Verification items for this drawing (mm, ordinates from the low corner). A direction names the side the tool comes from. Coordinates: 2 decimals unless noted, no trailing zeros. Order: outer loops, then holes, each group sorted by start corner. A loop starts at its lowest first (then second) coordinate and runs counter-clockwise, first axis right, second up. Notation, with made-up numbers: (-29, -5.75) - (-8, -5.75) arc R30 cw to (-8, 32.25) - close; hole circle Ø4 at (-24.5, 65). An arc over 180 degrees is marked (long way). Use CSV: the item, a comma, the result in double quotes. Start each with the question number.
1) Draft check along X on the marked faces 3, 4 and 5. Enter one of: released by +X, released by -X, zero draft, split by the parting line, or undercut.
2) Depth check by flat-ended pin: P1, Ø2.5, axis at y = 13.5, z = 11, coming from the -X side; P2, Ø5, axis at x = 10.5, y = 13, coming from the +Z side; P3, Ø1, axis at x = 16, y = 9, coming from the +Z side; P4, Ø2, axis at x = 18, z = 9, coming from the -Y side. Enter the tip coordinate at first touch or a pass-through.
3) Thickness scan on probe 1 along Y at (x, z) = (23.75, 7.5); probe 2 along Z at (x, y) = (23.75, 7.4); probe 3 along Y at (x, z) = (25, 7.75) (1 decimal). Record the ranges inside material, lowest first. Write a range as [from, to].
4) Sectioned sample at B-B, the plane z = 7.75. Record the cut outline in (x, y), and give its area (3 significant figures).
5) Tool access check on the marked faces 1 and 2. Record the directions out of +Z, -Z, +X, -X, +Y, -Y that give a thin tool (end or side, any length) a straight path to the whole face; none if there is none.
6) Sectioned sample at D-D, the plane z = 11.75. Record the cut outline in (x, y).
7) Sectioned sample at A-A, the plane x = 23.75. Record the cut outline in (y, z), and give its area (3 significant figures).
8) Sectioned sample at C-C, the plane y = 18.5. Record the cut outline in (x, z).
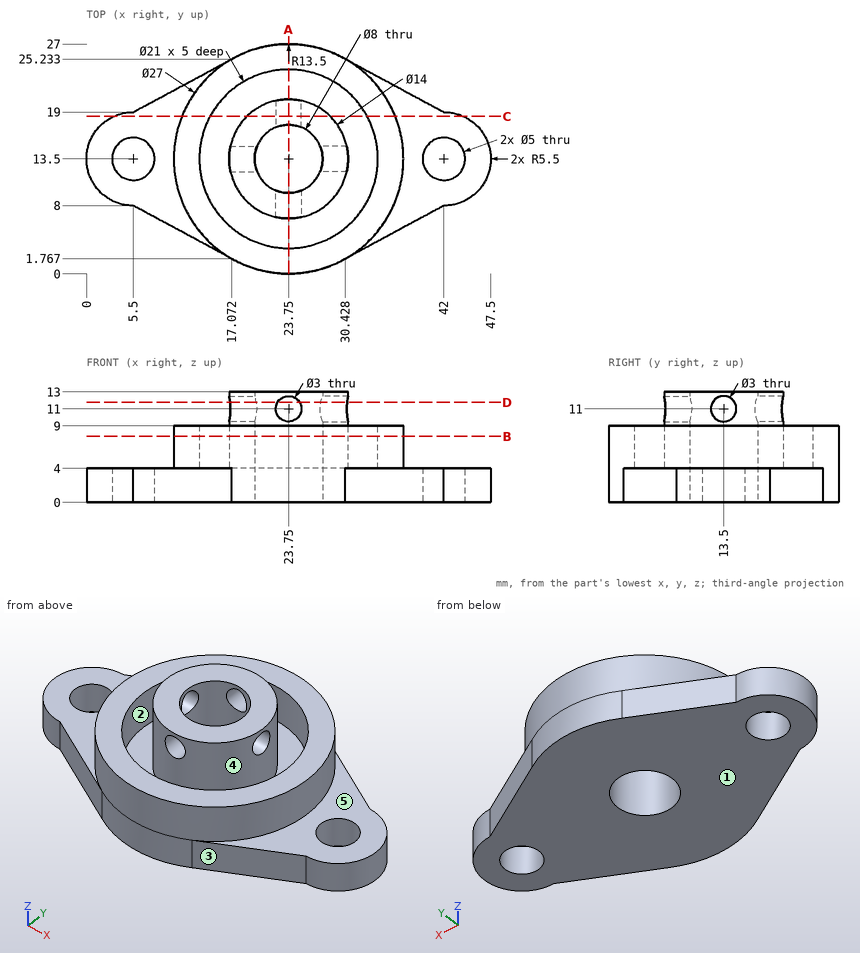
Evaluation:
1,face 3,"released by +X"
1,face 4,"undercut"
1,face 5,"zero draft"
2,P1,"through"
2,P2,"z = 9"
2,P3,"z = 4"
2,P4,"y = 0.86"
3,probe 1,"[0, 3], [6.5, 9.5], [17.5, 20.5], [24, 27]"
3,probe 2,"[0, 9.5], [12.5, 13]"
3,probe 3,"[0.1, 3.1], [6.6, 9.7], [17.3, 20.4], [23.9, 26.9]"
4,outline,"circle Ø27 at (23.75, 13.5); circle Ø14 at (23.75, 13.5); hole circle Ø21 at (23.75, 13.5); hole circle Ø8 at (23.75, 13.5)"
4,area,"330 mm²"
5,face 1,"-Z, +X, -X, +Y, -Y"
5,face 2,"+Z"
6,outline,"(16.87, 12.2) arc R7 ccw to (22.45, 6.62) - (22.45, 9.72) arc R4 cw to (19.97, 12.2) - close; (16.87, 14.8) - (19.97, 14.8) arc R4 cw to (22.45, 17.28) - (22.45, 20.38) arc R7 ccw to start; (25.05, 6.62) arc R7 ccw to (30.63, 12.2) - (27.53, 12.2) arc R4 cw to (25.05, 9.72) - close; (25.05, 17.28) arc R4 cw to (27.53, 14.8) - (30.63, 14.8) arc R7 ccw to (25.05, 20.38) - close"
7,outline,"(0, 0) - (9.5, 0) - (9.5, 9.5) - (6.5, 9.5) - (6.5, 4) - (3, 4) - (3, 9) - (0, 9) - close; (6.5, 12.5) - (9.5, 12.5) - (9.5, 13) - (6.5, 13) - close; (17.5, 0) - (27, 0) - (27, 9) - (24, 9) - (24, 4) - (20.5, 4) - (20.5, 9.5) - (17.5, 9.5) - close; (17.5, 12.5) - (20.5, 12.5) - (20.5, 13) - (17.5, 13) - close"
7,area,"142 mm²"
8,outline,"(3.21, 0) - (44.29, 0) - (44.29, 4) - (36.29, 4) - (36.29, 9) - (32.98, 9) - (32.98, 4) - (28.65, 4) - (28.65, 13) - (18.85, 13) - (18.85, 4) - (14.52, 4) - (14.52, 9) - (11.21, 9) - (11.21, 4) - (3.21, 4) - close; hole circle Ø3 at (23.75, 11)"
